Geometry check sheet. Reference: the model listing, model coordinates, mm. A direction names the side the tool comes from. Coordinates: 2 decimals unless noted, no trailing zeros. Order: outer loops, then holes, each group sorted by start corner. A loop starts at its lowest first (then second) coordinate and runs counter-clockwise, first axis right, second up. Notation, with made-up numbers: M 38.5,51 L 53.5,51 A16 cw 53.5,58 Z; hole C 29,72 d7. An arc over 180 degrees is marked long. One line per item, written item: value. Start each with the question number.
1) Draft check along Y on faces 3 (the flat face through (9.287, 79.111, 1.972)), 4 (the cylindrical face through (45.17, 8.86, 1.97)), 5 (the flat face through (4, 30, 4)), 6 (the flat face through (-8.8, 30.975, 1.972)). Enter one of: pulls with the +Y half, pulls with the -Y half, needs draft (parallel to the pull), parting line crosses it, or undercut.
2) Thickness scan on L1, parallel to Y at x = 16.5, z = 2.8; L2, parallel to X at y = -9.5, z = 2.35; L3, parallel to Y at x = -7.5, z = 0.95. Record the ranges inside material, lowest first. Write a range as from..to.
3) Sectioned sample at B-B, the plane z = 2.75. State how many separate pieces and enclosed holes the cut face has, then the cut area to 3 significant figures.
4) Sectioned sample at A-A, the plane x = -7. Enter the section's corners in (y, z).
5) Go/stop test with flat-tipped pins: P1, Ø1, axis at y = 56, z = 1.5, coming from the +X side; P2, Ø1.5, axis at x = -22.5, z = 3, coming from the -Y side; P3, Ø2, axis at x = 32.5, z = 1, coming from the -Y side. Record where each tip stops, or that it passes through.
6) Access from +Z, -Z, +X, -X, +Y, -Y to the whole of each face (thin tool, end or side, straight path). Record for faces 1 (the flat face through (32.271, -8, 2)), 2 (the flat face through (27.4, 72.25, 1.97)).
7) Sectioned sample at C-C, the plane y = 5. Enter the section's corners in (x, z), then the cut area to 3 significant figures.
```python
from build123d import *

# Parameters (mm, degrees)
SKETCH1_R           = 2
SKETCH1_R_2         = 3.5
SKETCH1_W           = 9.000072
SKETCH1_H           = 2
SKETCH1_W_2         = 5
BOSS_EXTRUDE1_DEPTH = 4
SKETCH2_W           = 8
SKETCH2_H           = 4
CUT_EXTRUDE1_DEPTH  = 96.21167482


with BuildPart() as part:
    # Sketch1 → Boss-Extrude1 (new body)
    with BuildSketch(Plane.XY):
        with BuildLine():
            Line((-12.978640908, -18), (-12.978640908, -24))
            Line((-12.978640908, -24), (23.021359092, -24))
            Line((23.021359092, -24), (23.021359092, -18))
            ThreePointArc((23.021359092, -18), (32.58126188, -15.140073441), (39, -7.5))
            ThreePointArc((39, -7.5), (45.227131985, 9.097629123), (47.343034567, 26.698237678))
            ThreePointArc((47.343034567, 26.698237678), (46.561018226, 46.955835458), (44.219623828, 67.092858318))
            Line((44.219623828, 67.092858318), (28.140376172, 69.067141682))
            Line((28.140376172, 69.067141682), (26.638766331, 75.523635508))
            Line((26.638766331, 75.523635508), (10.441233669, 75.806364492))
            Line((10.441233669, 75.806364492), (8.1, 82.51))
            Line((8.1, 82.51), (-8.1, 82.51))
            Line((-8.1, 82.51), (-14.491217975, 82.280462515))
            Line((-14.491217975, 82.280462515), (-30.688782025, 81.999537485))
            ThreePointArc((-30.688782025, 81.999537485), (-37.567707395, 47.245827753), (-37.052658257, 11.821617405))
            ThreePointArc((-37.052658257, 11.821617405), (-29.300451665, -6.548172019), (-12.978640908, -18))
        make_face()
        with Locations((38.147341743, 11.821617405)):
            Circle(SKETCH1_R, mode=Mode.SUBTRACT)
        with Locations((-24.678960076, 61.651218734)):
            Circle(SKETCH1_R_2, mode=Mode.SUBTRACT)
        with Locations(Location((1.521420673, 61.651218734, 0), (0, 0, 180))):
            Circle(SKETCH1_R_2, mode=Mode.SUBTRACT)
        with Locations((14.86306514, 46.821617405)):
            Circle(SKETCH1_R_2, mode=Mode.SUBTRACT)
        with Locations(Location((38.147341743, 46.821617405, 0), (0, 0, 180))):
            Circle(SKETCH1_R_2, mode=Mode.SUBTRACT)
        with Locations((-31.681501662, 43.456405989)):
            Circle(SKETCH1_R, mode=Mode.SUBTRACT)
        with Locations((0, 77.51)):
            Rectangle(SKETCH1_W, SKETCH1_H, mode=Mode.SUBTRACT)
        Polygon((-4, -2.5), (0, -2.5), (0, 0), (12, 0), (12, -2.5), (16, -2.5), (16, -12.5), (12, -12.5), (12, -15), (0, -15), (0, -12.5), (-4, -12.5), align=None, mode=Mode.SUBTRACT)
        with Locations((35.147341743, 56.321617405)):
            Rectangle(SKETCH1_W_2, SKETCH1_H, mode=Mode.SUBTRACT)
        Polygon((-27.019995137, 78.062566115), (-18.021276454, 78.218636824), (-17.986594351, 76.218937559), (-26.985313034, 76.062866849), align=None, mode=Mode.SUBTRACT)
        with Locations((17.86306514, 56.321617405)):
            Rectangle(SKETCH1_W_2, SKETCH1_H, mode=Mode.SUBTRACT)
        with Locations((-0.478579327, 71.151218734)):
            Rectangle(SKETCH1_W_2, SKETCH1_H, mode=Mode.SUBTRACT)
        Polygon((13.970839752, 71.744145677), (13.935934939, 69.744450286), (22.934636184, 69.587377372), (22.969540997, 71.587072762), align=None, mode=Mode.SUBTRACT)
        Polygon((40.15901604, 63.561398961), (31.226029212, 64.658231826), (30.982290526, 62.673139523), (39.915277354, 61.576306658), align=None, mode=Mode.SUBTRACT)
        Polygon((1.632632483, 35.912105076), (1.005748572, 29.944943559), (-18.884789816, 32.034556594), (-18.257905905, 38.00171811), align=None, mode=Mode.SUBTRACT)
        with Locations((-22.678960076, 71.151218734)):
            Rectangle(SKETCH1_W_2, SKETCH1_H, mode=Mode.SUBTRACT)
        Polygon((0.065422707, 20.994201285), (-1.188345114, 9.059878252), (-21.078883502, 11.149491286), (-19.825115681, 23.083814319), align=None, mode=Mode.SUBTRACT)
        Polygon((-9.666, 24.072796069), (-9.153, 28.955923243), (-23.205665371, 30.432234852), (-22.787742764, 34.410342529), (-30.743958119, 35.246187743), (-31.161880726, 31.268080066), (-34.143965433, 31.581364852), (-34.656965433, 26.698237678), (-31.674880726, 26.384952891), (-32.092803333, 22.406845214), (-24.136587978, 21.571), (-23.718665371, 25.549107678), align=None, mode=Mode.SUBTRACT)
    extrude(amount=BOSS_EXTRUDE1_DEPTH)

    # Sketch2 → Cut-Extrude1 (cut, through all)
    with BuildSketch(Plane(origin=(0, 0, 0), x_dir=(-1, 0, 0), z_dir=(0, 0, -1))):
        with Locations((-28.271359092, -8)):
            Rectangle(SKETCH2_W, SKETCH2_H)
        with Locations((18.228640908, -8)):
            Rectangle(SKETCH2_W, SKETCH2_H)
    extrude(amount=-CUT_EXTRUDE1_DEPTH, mode=Mode.SUBTRACT)


solid = part.part
```
Final values:
1. face 3: pulls with the +Y half
1. face 4: pulls with the -Y half
1. face 5: needs draft
1. face 6: undercut
2. L1: y = -24..43.73, 49.92..55.32, 57.32..69.7, 71.7..75.7
2. L2: x = -26.64..-22.23, -14.23..-4, 16..24.27, 32.27..37.98
2. L3: y = -24..9.72, 21.79..30.84, 36.87..82.51
3. separate pieces: 1
3. enclosed holes: 20
3. area: 6,580 mm^2
4. outline: M -24,0 L 9.67,0 L 9.67,4 L -24,4 Z; M 21.74,0 L 30.79,0 L 30.79,4 L 21.74,4 Z; M 36.82,0 L 82.51,0 L 82.51,4 L 36.82,4 Z
5. P1: stops at x = 45.76
5. P2: stops at y = -13.56
5. P3: stops at y = -15.8
6. face 1: +Z, -Z
6. face 2: +Z, -Z, +X, +Y
7. outline: M -35.55,0 L 44.1,0 L 44.1,4 L -35.55,4 Z
7. area: 319 mm^2
